```python
from build123d import *

# Parameters (mm, degrees)
CROQUIS1_R              = 3.5
SALIENTE_EXTRUIR1_DEPTH = 8
CROQUIS2_R              = 3.5
SALIENTE_EXTRUIR2_DEPTH = 1
CROQUIS3_R              = 3.5
SALIENTE_EXTRUIR3_DEPTH = 10


with BuildPart() as part:
    # Croquis1 → Saliente-Extruir1 (new body)
    with BuildSketch(Plane.XY):
        with Locations((-55.120752438, 48.948230875)):
            Circle(CROQUIS1_R)
        with BuildLine():
            Line((-55.570752438, 46.489064349), (-55.570752438, 47.089064349))
            Line((-55.570752438, 47.089064349), (-54.670752438, 47.089064349))
            Line((-54.670752438, 47.089064349), (-54.670752438, 46.489064349))
            ThreePointArc((-54.670752438, 46.489064349), (-55.120752438, 51.448230875), (-55.570752438, 46.489064349))
        make_face(mode=Mode.SUBTRACT)
    extrude(amount=SALIENTE_EXTRUIR1_DEPTH)

    # Croquis2 → Saliente-Extruir2 (add)
    with BuildSketch(Plane.XY.offset(8)):
        with Locations((-55.120752438, 48.948230875)):
            Circle(CROQUIS2_R)
    extrude(amount=SALIENTE_EXTRUIR2_DEPTH)

    # Croquis3 → Saliente-Extruir3 (add)
    with BuildSketch(Plane.XY.offset(9)):
        with Locations((-55.120752438, 48.948230875)):
            Circle(CROQUIS3_R)
        with BuildLine():
            Line((-55.570752438, 51.4073974), (-55.570752438, 52.0073974))
            Line((-55.570752438, 52.0073974), (-54.670752438, 52.0073974))
            Line((-54.670752438, 52.0073974), (-54.670752438, 51.4073974))
            ThreePointArc((-54.670752438, 51.4073974), (-55.120752438, 46.448230875), (-55.570752438, 51.4073974))
        make_face(mode=Mode.SUBTRACT)
    extrude(amount=SALIENTE_EXTRUIR3_DEPTH)


solid = part.part
```
CAD build for the part. Positions are in the model's coordinates, mm. A direction names the side the tool comes from. Coordinates: 2 decimals unless noted, no trailing zeros. Loops run counter-clockwise (first coordinate to the right, second up) from the corner with the lowest first, then second, coordinate; pieces in that order, holes last. Notation, with made-up numbers: (5.5, 57.25) - (44.5, 57.25) arc R23 cw to (44.5, 65.25) - close; hole circle Ø8 at (46, 62.5). An arc over 180 degrees is marked (long way). Return JSON: item names as keys, results as strings.
1. Band-saw the part on D-D (z = 14.25). Give the cut face in (x, y), and give its area (3 significant figures).
Result:
{"outline": "circle Ø7 at (-55.12, 48.95); hole (-55.57, 51.41) arc R2.5 ccw (long way) to (-54.67, 51.41) - (-54.67, 52.01) - (-55.57, 52.01) - close", "area": "18.3 mm2"}
2. Band-saw the part on A-A (z = 2.5). Give the cut face in (x, y), and give its area (3 significant figures).
Result:
{"outline": "circle Ø7 at (-55.12, 48.95); hole (-55.57, 46.49) - (-55.57, 47.09) - (-54.67, 47.09) - (-54.67, 46.49) arc R2.5 ccw (long way) to start", "area": "19.4 mm2"}
3. Probe L1, parallel to Z at x = -54.75, y = 49.75; L2, parallel to X at y = 49, z = 13.5; L3, parallel to X at y = 51, z = 15.75. List the from-to ranges inside material, lowest first. Write a range as from..to.
Result:
{"L1": "z = 8..9", "L2": "x = -58.62..-57.62, -52.62..-51.62", "L3": "x = -57.96..-56.55, -53.69..-52.29"}
4. Mould opens along Y. For faces 1 (the flat face through (-58, 50, 19)), 2 (the flat face through (-55, 52.007, 14)), 3 (the cylindrical face through (-51.888, 47.608, 9.367)) say: released by +Y, released by -Y, zero draft, split by the parting line, or undercut.
Result:
{"face 1": "zero draft", "face 2": "undercut", "face 3": "split by the parting line"}
5. Band-saw the part on C-C (y = 47.5). Give the cut face in (x, z).
Result:
{"outline": "(-58.31, 0) - (-57.16, 0) - (-57.16, 8) - (-53.08, 8) - (-53.08, 0) - (-51.93, 0) - (-51.93, 19) - (-53.08, 19) - (-53.08, 9) - (-57.16, 9) - (-57.16, 19) - (-58.31, 19) - close"}
6. 3-axis set-ups, long thin cutter, end or side, ignore diameter. For faces 4 (the flat face through (-55, 47.089, 4)), 5 (the flat face through (-55, 49, 9)), 6 (the flat face through (-55.2, 46.7, 0)): which of +Z, -Z, +X, -X, +Y, -Y reach the whole face in a straight line?
Result:
{"face 4": "-Z", "face 5": "+Z", "face 6": "-Z, +X, -X, +Y, -Y"}
7. Drop flat-ended pins along their axis: pin 1 (2.5 mm diameter, centred on x = -55.5, y = 50, fed in from -Z); pin 2 (1 mm diameter, centred on x = -56, z = 12.5, fed in from +Y); pin 3 (3 mm diameter, centred on x = -58, z = 16.5, fed in from -Y); pin 4 (4 mm diameter, centred on x = -54, y = 49.5, fed in from +Z). Give the stop position or say it passes through.
Result:
{"pin 1": "stops at z = 8", "pin 2": "stops at y = 52.43", "pin 3": "stops at y = 45.73", "pin 4": "stops at z = 19"}
8. Band-saw the part on B-B (x = -54). Give the cut face in (y, z).
Result:
{"outline": "(45.63, 0) - (46.71, 0) - (46.71, 8) - (51.18, 8) - (51.18, 0) - (52.26, 0) - (52.26, 19) - (51.18, 19) - (51.18, 9) - (46.71, 9) - (46.71, 19) - (45.63, 19) - close"}
